Can you work these out from the model? Positions are in its coordinate system, mm. A direction names the side the tool comes from. Round coordinates to 2 decimals unless told otherwise and drop trailing zeros. Loops run counter-clockwise (first coordinate to the right, second up) from the corner with the lowest first, then second, coordinate; pieces in that order, holes last. Notation, with made-up numbers: (-4, 51) -> (24, 51) arc R26 ccw to (24, 84) -> close; hole circle Ø9 at (63.25, 34). An arc over 180 degrees is marked (long way). Write each question's results on one line, items separated by ' | '.
from build123d import *

# Parameters (mm, degrees)
BOSS_EXTRUDE1_DEPTH = 42.5


with BuildPart() as part:
    # Sketch1 → Boss-Extrude1 (new, symmetric)
    with BuildSketch(Plane(origin=(0, 0, 0), x_dir=(1, 0, 0), z_dir=(0, 1, 0))):
        with BuildLine():
            Line((-43.393852632, -25.264521876), (-59.645031086, 13.969293553))
            ThreePointArc((-59.645031086, 13.969293553), (-59.576188638, 17.954532916), (-56.615582649, 20.623181309))
            ThreePointArc((-56.615582649, 20.623181309), (0.444031685, 29.937093688), (57.50364602, 20.623181309))
            ThreePointArc((57.50364602, 20.623181309), (60.464252009, 17.954532916), (60.533094457, 13.969293553))
            Line((60.533094457, 13.969293553), (44.281916002, -25.264521876))
            ThreePointArc((44.281916002, -25.264521876), (41.909163826, -27.81793626), (38.444552916, -28.200492328))
            ThreePointArc((38.444552916, -28.200492328), (0.444031685, -23.501385869), (-37.556489545, -28.200492328))
            ThreePointArc((-37.556489545, -28.200492328), (-41.021100455, -27.81793626), (-43.393852632, -25.264521876))
        make_face()
        with BuildLine():
            Line((-26.579395894, -0.530063133), (-27.767590131, 2.338491509))
            ThreePointArc((-27.767590131, 2.338491509), (0.444031685, 4.937093688), (28.655653502, 2.338491509))
            Line((28.655653502, 2.338491509), (27.467459265, -0.530063133))
            ThreePointArc((27.467459265, -0.530063133), (0.444031685, 1.498614131), (-26.579395894, -0.530063133))
        make_face(mode=Mode.SUBTRACT)
    extrude(amount=BOSS_EXTRUDE1_DEPTH, both=True)


solid = part.part
1. If we section it at D-D (z = 20.5): List the corners of the cut face in (x, y) for me, then the cut area to 3 significant figures.
Final values:
outline: (-45.37, -42.5) -> (46.26, -42.5) -> (46.26, 42.5) -> (-45.37, 42.5) -> close | area: 7,790 mm2
2. Please list where these lines run through material, in increasing order: line 1 (Z direction, x = 26.5, y = 7); line 2 (Z direction, x = -11, y = 30); line 3 (Z direction, x = -50, y = -32). Write a range as from..to.
Final values:
line 1: -28.04..-2.72, 0.39..25.69 | line 2: -29.57..-4.51, -1.14..23.92 | line 3: -22.7..9.32
3. If we section it at C-C (x = 15): List the corners of the cut face in (y, z) for me, then the cut area to 3 significant figures.
Final values:
outline: (-42.5, -29.35) -> (42.5, -29.35) -> (42.5, -4.25) -> (-42.5, -4.25) -> close; (-42.5, -0.91) -> (42.5, -0.91) -> (42.5, 24.18) -> (-42.5, 24.18) -> close | area: 4,270 mm2
4. Will these pins go through, and if not, where does the flat tip stop? pin 1 (3 mm diameter, centred on y = -1, z = -2, fed in from +X); pin 2 (8 mm diameter, centred on y = -18, z = 8, fed in from -X); pin 3 (4 mm diameter, centred on y = -23, z = 14, fed in from +X).
Final values:
pin 1: x = 56.2 | pin 2: x = -52.2 | pin 3: x = 49.78
5. On a 3-axis mill with a long thin cutter (end or side, diameter ignored), from which of +Z, -Z, +X, -X, +Y, -Y can I reach the whole of each face in a straight line? I mean faces 1 (the face through (-27.165, 0.595, -0.884)), 2 (the face through (60.44, 0.59, -18.01)). Say none if no direction works.
Final values:
face 1: +Y, -Y | face 2: +X, +Y, -Y
6. We'd pull the mould along X, two halves only. Please class faces 3 (the face through (0.047, 0.595, -4.937)), 4 (the face through (28.07, 0.59, -0.92)), 5 (the face through (-51.406, 0.595, 5.922)), 6 (the face through (1, -42.5, -1)): pulls with the +X half, pulls with the -X half, needs draft (parallel to the pull), parting line crosses it, or undercut.
Final values:
face 3: undercut | face 4: undercut | face 5: pulls with the -X half | face 6: needs draft
7. If we section it at A-A (x = -9): List the corners of the cut face in (y, z) for me, then the cut area to 3 significant figures.
Final values:
outline: (-42.5, -29.69) -> (42.5, -29.69) -> (42.5, -4.65) -> (-42.5, -4.65) -> close; (-42.5, -1.25) -> (42.5, -1.25) -> (42.5, 23.79) -> (-42.5, 23.79) -> close | area: 4,260 mm2
8. If we section it at B-B (y = -32.5): List the corners of the cut face in (x, z) for me, then the cut area to 3 significant figures.
Final values:
outline: (-59.65, -13.97) arc R5 ccw to (-56.62, -20.62) arc R179.44 ccw to (57.5, -20.62) arc R5 ccw to (60.53, -13.97) -> (44.28, 25.26) arc R5 ccw to (38.44, 28.2) arc R156 cw to (-37.56, 28.2) arc R5 ccw to (-43.39, 25.26) -> close; hole (-27.77, -2.34) arc R154.44 ccw to (28.66, -2.34) -> (27.47, 0.53) arc R181 cw to (-26.58, 0.53) -> close | area: 5,410 mm2
